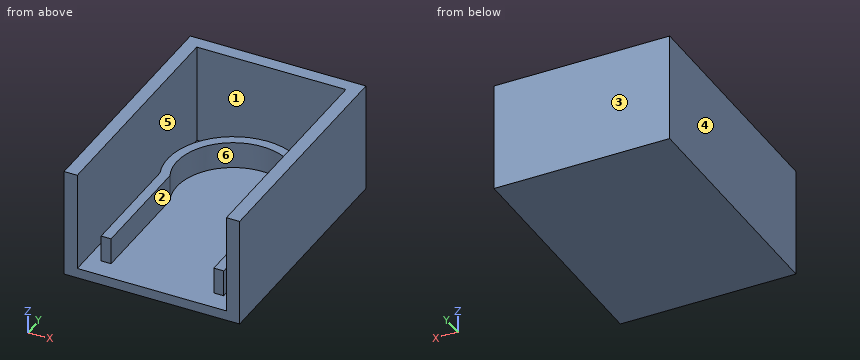
from build123d import *

# Parameters (mm, degrees)
BOSS_EXTRUDE1_DEPTH = 4
SKETCH3_W           = 22.5
SKETCH3_H           = 35
BOSS_EXTRUDE2_DEPTH = 1.5
BOSS_EXTRUDE5_DEPTH = 15
BOSS_EXTRUDE6_DEPTH = 1.5


with BuildPart() as part:
    # Sketch1 → Boss-Extrude1 (new body)
    with BuildSketch(Plane.XY):
        with BuildLine():
            Line((-7.75, -19.202403031), (-7.75, -3.491060011))
            ThreePointArc((-7.75, -3.491060011), (0, 8.5), (7.75, -3.491060011))
            Line((7.75, -3.491060011), (7.75, -19.202403031))
            Line((7.75, -19.202403031), (7.75, -20.702403031))
            Line((7.75, -20.702403031), (9.25, -20.702403031))
            Line((9.25, -20.702403031), (9.25, -3.491060011))
            ThreePointArc((9.25, -3.491060011), (0, 9.961709327), (-9.25, -3.491060011))
            Line((-9.25, -3.491060011), (-9.25, -20.702403031))
            Line((-9.25, -20.702403031), (-7.75, -20.702403031))
            Line((-7.75, -20.702403031), (-7.75, -19.202403031))
        make_face()
    extrude(amount=BOSS_EXTRUDE1_DEPTH)

    # Sketch3 → Boss-Extrude2 (add)
    with BuildSketch(Plane.XY):
        with Locations((0, -6.3)):
            Rectangle(SKETCH3_W, SKETCH3_H)
    extrude(amount=-BOSS_EXTRUDE2_DEPTH)



with BuildPart() as body_2:
    # Sketch9 → Boss-Extrude5 (new body)
    with BuildSketch(Plane.XY):
        Polygon((-13.25, 13.2), (13.25, 13.2), (13.25, -23.8), (11.25, -23.8), (11.25, 11.2), (-11.25, 11.2), (-11.25, -23.8), (-13.25, -23.8), align=None)
    extrude(amount=BOSS_EXTRUDE5_DEPTH)


with BuildPart() as part_1:
    add(part.part)

    add(body_2.part)  # Boss-Extrude6 merges body 2
    # Sketch10 → Boss-Extrude6 (add)
    with BuildSketch(Plane.XY):
        Polygon((-13.25, 13.2), (13.25, 13.2), (13.25, -23.8), (11.25, -23.8), (11.25, 11.2), (-11.25, 11.2), (-11.25, -23.8), (-13.25, -23.8), align=None)
    extrude(amount=-BOSS_EXTRUDE6_DEPTH)


solid = part_1.part
Read the model definition and answer for the solid it produces. Units are mm, in the model's axes. Face numbers are marked on the shaded views. A direction names the side the tool comes from. Coordinates: 2 decimals unless noted, no trailing zeros. Write each loop counter-clockwise with the first axis right and the second up, starting at its lowest first coordinate (ties: lowest second). Pieces come first, ordered by that corner, then holes. Notation, with made-up numbers: M 64,5.25 L 74,5.25 A16 cw 74,15.25 Z; hole C -12,49 d2. An arc over 180 degrees is marked long. Use a Markdown table: item, result.
Q1. Each of these flat-tipped pins is pushed along its axis until it touches: pin 1 Ø5 at (x, z) = (-3, 13) entering from -Y; pin 2 Ø4 at (x, y) = (6.5, 5) entering from +Z; pin 3 Ø1.6 at (x, z) = (-8.5, 1.5) entering from -Y. Where does it stop, or does it pass through?
Answer block:
| item | result |
|---|---|
| pin 1 | stops at y = 11.2 |
| pin 2 | stops at z = 4 |
| pin 3 | stops at y = -20.7 |
Q2. The part is cut by section D-D, the plane z = 5. Write down the section's boundary in (x, y), then the cut area to 3 significant figures.
Answer block:
| item | result |
|---|---|
| outline | M -13.25,-23.8 L -11.25,-23.8 L -11.25,11.2 L 11.25,11.2 L 11.25,-23.8 L 13.25,-23.8 L 13.25,13.2 L -13.25,13.2 Z |
| area | 193 mm2 |
Q3. The part is cut by section B-B, the plane y = -17. Write down the section's boundary in (x, z).
Answer block:
| item | result |
|---|---|
| outline | M -13.25,-1.5 L 13.25,-1.5 L 13.25,15 L 11.25,15 L 11.25,0 L 9.25,0 L 9.25,4 L 7.75,4 L 7.75,0 L -7.75,0 L -7.75,4 L -9.25,4 L -9.25,0 L -11.25,0 L -11.25,15 L -13.25,15 Z |
Q4. Determine the mould class of the marked faces 1, 2 and 3 for opening direction Y: released by +Y, released by -Y, zero draft, split by the parting line, or undercut.
Answer block:
| item | result |
|---|---|
| face 1 | undercut |
| face 2 | zero draft |
| face 3 | released by +Y |
Q5. Which of the six approach directions +Z, -Z, +X, -X, +Y, -Y give full straight-line access (tool end or side, diameter ignored) to the marked faces 4, 5 and 6?
Answer block:
| item | result |
|---|---|
| face 4 | +Z, -Z, -X, +Y, -Y |
| face 5 | +Z, -Y |
| face 6 | +Z |
Q6. The part is cut by section C-C, the plane x = -0.5. Write down the section's boundary in (y, z), then the cut area to 3 significant figures.
Answer block:
| item | result |
|---|---|
| outline | M -23.8,-1.5 L 13.2,-1.5 L 13.2,15 L 11.2,15 L 11.2,0 L 9.95,0 L 9.95,4 L 8.49,4 L 8.49,0 L -23.8,0 Z |
| area | 91.4 mm2 |
Q7. Straight lines are drawn through the part: L1, parallel to X at y = -19.5, z = 2.25; L2, parallel to X at y = 0, z = 2.8; L3, parallel to X at y = -19, z = 6.25. For each, find the intervals that lie inside material, in ascending order. Write a range as [from, to].
Answer block:
| item | result |
|---|---|
| L1 | x = [-13.25, -11.25], [-9.25, -7.75], [7.75, 9.25], [11.25, 13.25] |
| L2 | x = [-13.25, -11.25], [-9.91, -8.5], [8.5, 9.91], [11.25, 13.25] |
| L3 | x = [-13.25, -11.25], [11.25, 13.25] |
Q8. The part is cut by section A-A, the plane z = 3.25. Write down the section's boundary in (x, y), then the cut area to 3 significant figures.
Answer block:
| item | result |
|---|---|
| outline | M -13.25,-23.8 L -11.25,-23.8 L -11.25,11.2 L 11.25,11.2 L 11.25,-23.8 L 13.25,-23.8 L 13.25,13.2 L -13.25,13.2 Z; M -9.25,-20.7 L -7.75,-20.7 L -7.75,-3.49 A8.5 cw long 7.75,-3.49 L 7.75,-20.7 L 9.25,-20.7 L 9.25,-3.49 A9.91 ccw long -9.25,-3.49 Z |
| area | 296 mm2 |
